Geometry check sheet. Reference: the model listing, model coordinates, mm. A direction names the side the tool comes from. Round coordinates to 2 decimals unless told otherwise and drop trailing zeros. Write each loop counter-clockwise with the first axis right and the second up, starting at its lowest first coordinate (ties: lowest second). Pieces come first, ordered by that corner, then holes. Notation, with made-up numbers: M -2.5,-3.75 L 5.5,-3.75 A24 cw 5.5,31.25 Z; hole C -27,-32 d2. An arc over 180 degrees is marked long. One line per item, written item: value. Start each with the question number.
1. Section check C-C (y = 0). Record the boundary of the cut face in (x, z) (3 decimals).
2. Access from +Z, -Z, +X, -X, +Y, -Y to the whole of each face (thin tool, end or side, straight path). Record for faces 4 (the cylindrical face through (-28.548, 15.809, 17.612)), 5 (the flat face through (29, 9.4, 17)), 6 (the flat face through (-19, 3, 17)), 7 (the cylindrical face through (0.06, -13.231, 18.874)), 8 (the flat face through (-33, 16, 17)).
3. Section check B-B (z = 17.5). Record the boundary of the cut face in (x, y) (3 decimals).
4. Section check D-D (x = 26). Record the boundary of the cut face in (y, z), and give its area (3 significant figures).
5. Release check for a two-part mould opening along Z. For faces 1 (the flat face through (0, 22.4, 17)), 2 (the flat face through (0, 16, 0)), 3 (the cylindrical face through (23.452, 15.809, 17.612)) record: pulls with the +Z half, pulls with the -Z half, needs draft (parallel to the pull), parting line crosses it, or undercut.
6. Section check A-A (x = 0). Record the boundary of the cut face in (y, z) (3 decimals).
7. Scan lines: probe 1 along Z at (x, y) = (26, 15); probe 2 along Y at (x, z) = (0, 13) (3 decimals); probe 3 along Z at (x, y) = (0, -13) (3 decimals). Record each from-to range of solid material in increasing order. Write a range as [from, to].
8. Depth check by flat-ended pin: P1, Ø8, axis at x = -26, z = 17.5, coming from the -Y side; P2, Ø6.5, axis at y = 2.5, z = 23, coming from the -X side; P3, Ø19, axis at x = 0, y = 0, coming from the +Z side; P4, Ø12, axis at x = 18, z = 15, coming from the -Y side. Enter the tip coordinate at first touch or a pass-through.
from build123d import *

# Parameters (mm, degrees)
CROQUIS1_R                 = 10.475
SALIENTE_EXTRUIR1_DEPTH    = 35
CROQUIS2_R                 = 2.55
CORTAR_EXTRUIR1_DEPTH      = 55.398161734
CHAFL_N1_SIZE              = 2
CORTAR_EXTRUIR2_REACH      = 63.551
CORTAR_EXTRUIR2_END_RADIUS = 10.475
CROQUIS3_R                 = 1.375


with BuildPart() as part:
    # Croquis1 → Saliente-Extruir1 (new body)
    with BuildSketch(Plane.XY):
        with BuildLine():
            Line((-33, 22.4), (33, 22.4))
            Line((33, 22.4), (33, 9.4))
            Line((33, 9.4), (19, 9.4))
            Line((19, 9.4), (19, -4))
            ThreePointArc((19, -4), (15.485281374, -12.485281374), (7, -16))
            Line((7, -16), (-7, -16))
            ThreePointArc((-7, -16), (-15.485281374, -12.485281374), (-19, -4))
            Line((-19, -4), (-19, 9.4))
            Line((-19, 9.4), (-33, 9.4))
            Line((-33, 9.4), (-33, 22.4))
        make_face()
        Circle(CROQUIS1_R, mode=Mode.SUBTRACT)
    extrude(amount=SALIENTE_EXTRUIR1_DEPTH)

    # Croquis2 → Cortar-Extruir1 (cut, through all)
    with BuildSketch(Plane.XZ.offset(-9.4)):
        with Locations((-26, 17.5)):
            Circle(CROQUIS2_R)
        with Locations((26, 17.5)):
            Circle(CROQUIS2_R)
    extrude(amount=-CORTAR_EXTRUIR1_DEPTH, mode=Mode.SUBTRACT)

    # Chaflán1
    chafl_n1_edges = [part.edges().sort_by_distance(p)[0] for p in [
        (-10.475, 0, 0),
        (-10.475, 0, 35),
    ]]
    chamfer(chafl_n1_edges, length=CHAFL_N1_SIZE)

    # Cortar-Extruir2: up to this cylinder (the profile starts outside it)
    cortar_extruir2_end = Plane(origin=(0, 0, 17.5), z_dir=(0, 0, -1)) * Cylinder(CORTAR_EXTRUIR2_END_RADIUS, 149.052, mode=Mode.PRIVATE)
    # Croquis3 → Cortar-Extruir2 (cut, up to the surface)
    with BuildSketch(Plane.XZ.offset(16), mode=Mode.PRIVATE) as cortar_extruir2_sk1:
        with Locations(Location((0, 17.5, 0), (0, 0, 270))):
            Circle(CROQUIS3_R)
    cortar_extruir2_tool1 = extrude(cortar_extruir2_sk1.sketch, amount=-CORTAR_EXTRUIR2_REACH, mode=Mode.PRIVATE) - cortar_extruir2_end
    add(cortar_extruir2_tool1.solids().sort_by_distance((0, -16, 17.5))[0], mode=Mode.SUBTRACT)


solid = part.part
Result sheet:
1. outline: M -19,0 L -12.475,0 L -10.475,2 L -10.475,33 L -12.475,35 L -19,35 Z; M 10.475,2 L 12.475,0 L 19,0 L 19,35 L 12.475,35 L 10.475,33 Z
2. face 4: +Y, -Y
2. face 5: +Z, -Z, +X, -Y
2. face 6: +Z, -Z, -X, -Y
2. face 7: -Y
2. face 8: +Z, -Z, -X, +Y, -Y
3. outline: M -33,9.4 L -28.55,9.4 L -28.55,22.4 L -33,22.4 Z; M -23.45,9.4 L -19,9.4 L -19,-4 A12 ccw -7,-16 L -1.375,-16 L -1.375,-10.384 A10.475 cw long 1.375,-10.384 L 1.375,-16 L 7,-16 A12 ccw 19,-4 L 19,9.4 L 23.45,9.4 L 23.45,22.4 L -23.45,22.4 Z; M 28.55,9.4 L 33,9.4 L 33,22.4 L 28.55,22.4 Z
4. outline: M 9.4,0 L 22.4,0 L 22.4,14.95 L 9.4,14.95 Z; M 9.4,20.05 L 22.4,20.05 L 22.4,35 L 9.4,35 Z
4. area: 389 mm2
5. face 1: needs draft
5. face 2: pulls with the -Z half
5. face 3: undercut
6. outline: M -16,0 L -12.475,0 L -10.475,2 L -10.475,16.125 L -16,16.125 Z; M -16,18.875 L -10.475,18.875 L -10.475,33 L -12.475,35 L -16,35 Z; M 10.475,2 L 12.475,0 L 22.4,0 L 22.4,35 L 12.475,35 L 10.475,33 Z
7. probe 1: z = [0, 14.95], [20.05, 35]
7. probe 2: y = [-16, -10.475], [10.475, 22.4]
7. probe 3: z = [0, 16.125], [18.875, 35]
8. P1: stops at y = 9.4
8. P2: stops at x = -19
8. P3: passes through
8. P4: stops at y = -14.91
